The listing builds one solid part. Answer for the finished solid, in the listing's coordinates (mm). Round coordinates to 2 decimals unless told otherwise and drop trailing zeros. Write each loop counter-clockwise with the first axis right and the second up, starting at its lowest first coordinate (ties: lowest second). Pieces come first, ordered by that corner, then holes. Notation, with made-up numbers: (75.5, 82.25) - (101.5, 82.25) arc R22 ccw to (101.5, 89.25) - close; hole circle Ø5 at (61, 30.5). An arc over 180 degrees is marked (long way). Answer in a Markdown table with one row per item.
from build123d import *

# Parameters (mm, degrees)
SKETCH3_R           = 19.05
BOSS_EXTRUDE1_DEPTH = 25.4
SKETCH4_R           = 3.81
CUT_EXTRUDE1_DEPTH  = 25.4
FILLET1_R           = 2.54


with BuildPart() as part:
    # Sketch3 → Boss-Extrude1 (new body)
    with BuildSketch(Plane(origin=(0, 0, 0), x_dir=(1, 0, 0), z_dir=(0, 1, 0))):
        with Locations(Location((0, 0, 0), (0, 0, 270))):
            Circle(SKETCH3_R)
    extrude(amount=BOSS_EXTRUDE1_DEPTH)

    # Sketch4 → Cut-Extrude1 (cut)
    with BuildSketch(Plane(origin=(0, 25.4, 0), x_dir=(1, 0, 0), z_dir=(0, 1, 0))):
        with Locations(Location((0, 0, 0), (0, 0, 270))):
            Circle(SKETCH4_R)
    extrude(amount=-CUT_EXTRUDE1_DEPTH, mode=Mode.SUBTRACT)

    # Fillet1
    fillet1_edges = [part.edges().sort_by_distance(p)[0] for p in [
        (0, 25.4, -19.05),
        (0, 0, -3.81),
        (0, 25.4, -3.81),
    ]]
    fillet(fillet1_edges, radius=FILLET1_R)


solid = part.part
(1) Section C-C (y = 10) is taken. Give the vertices of the cut face in (x, z), and give its area (3 significant figures).
Checked values:
| item | result |
|---|---|
| outline | circle Ø38.1 at (0, 0); hole circle Ø7.62 at (0, 0) |
| area | 1,090 mm2 |
(2) Section D-D (y = 23.5) is taken. Give the vertices of the cut face in (x, z).
Checked values:
| item | result |
|---|---|
| outline | circle Ø37.94 at (0, 0); hole circle Ø7.78 at (0, 0) |
(3) For a pull along X with two mould halves and no side action, classify faces 1 (the flat face through (-7, 25.4, 0)), 2 (the cylindrical face through (3.778, 12.842, -0.496)), 3 (the cylindrical face through (-11.59, 11.27, -15.12)) as pulls with the +X half, pulls with the -X half, needs draft (parallel to the pull), parting line crosses it, or undercut.
Checked values:
| item | result |
|---|---|
| face 1 | needs draft |
| face 2 | undercut |
| face 3 | parting line crosses it |
(4) Find the intervals of material crossed by line 1 (X direction, y = 17.25, z = 0); line 2 (Z direction, x = 3.5, y = 7.75); line 3 (X direction, y = 9, z = -2.5), in increasing order.
Checked values:
| item | result |
|---|---|
| line 1 | x = -19.05 to -3.81, 3.81 to 19.05 |
| line 2 | z = -18.73 to -1.51, 1.51 to 18.73 |
| line 3 | x = -18.89 to -2.88, 2.88 to 18.89 |
(5) Flat-ended cylindrical pins translate along their axes: pin 1 (3 mm diameter, centred on y = 18.5, z = 6.5, fed in from -X); pin 2 (5 mm diameter, centred on y = 17, z = -2, fed in from -X); pin 3 (1.5 mm diameter, centred on x = 0.5, y = 12, fed in from +Z); pin 4 (8 mm diameter, centred on x = -11, y = 16.5, fed in from +Z). Find the tip coordinate at first contact, or state that the pin passes through.
Checked values:
| item | result |
|---|---|
| pin 1 | stops at x = -18.38 |
| pin 2 | stops at x = -19.05 |
| pin 3 | stops at z = 19.05 |
| pin 4 | stops at z = 17.72 |
(6) Section B-B (z = 0) is taken. Give the vertices of the cut face in (x, y), and give its area (3 significant figures).
Checked values:
| item | result |
|---|---|
| outline | (-19.05, 0) - (-6.35, 0) arc R2.54 ccw to (-3.81, 2.54) - (-3.81, 22.86) arc R2.54 ccw to (-6.35, 25.4) - (-16.51, 25.4) arc R2.54 ccw to (-19.05, 22.86) - close; (3.81, 2.54) arc R2.54 ccw to (6.35, 0) - (19.05, 0) - (19.05, 22.86) arc R2.54 ccw to (16.51, 25.4) - (6.35, 25.4) arc R2.54 ccw to (3.81, 22.86) - close |
| area | 766 mm2 |
(7) Section A-A (x = 0) is taken. Give the vertices of the cut face in (y, z), and give its area (3 significant figures).
Checked values:
| item | result |
|---|---|
| outline | (0, -19.05) - (22.86, -19.05) arc R2.54 ccw to (25.4, -16.51) - (25.4, -6.35) arc R2.54 ccw to (22.86, -3.81) - (2.54, -3.81) arc R2.54 ccw to (0, -6.35) - close; (0, 6.35) arc R2.54 ccw to (2.54, 3.81) - (22.86, 3.81) arc R2.54 ccw to (25.4, 6.35) - (25.4, 16.51) arc R2.54 ccw to (22.86, 19.05) - (0, 19.05) - close |
| area | 766 mm2 |
